```python
from build123d import *

# Parameters (mm, degrees)
SKETCH_1_W          = 250
SKETCH_1_H          = 4
EXTRUDE_1_DEPTH     = 20
EXTRUDE_1_2_DEPTH   = 20
SKETCH_2_W          = 250
SKETCH_2_H          = 28
EXTRUDE_2_DEPTH     = 4
SKETCH_3_W          = 250
SKETCH_3_H          = 4
EXTRUDE_3_DEPTH     = 48.5
EXTRUDE_4_DEPTH     = 250
CUT_EXTRUDE_1_DEPTH = 55
FILLET_1_R          = 2
CUT_EXTRUDE_2_DEPTH = 250


with BuildPart() as part:
    # Sketch 1 → Extrude 1 (new body)
    with BuildSketch(Plane(origin=(0, 0, 0), x_dir=(0, 0, -1), z_dir=(1, 0, 0))):
        with Locations((84.36416185, 14.963552055)):
            Rectangle(SKETCH_1_W, SKETCH_1_H)
    extrude(amount=EXTRUDE_1_DEPTH)



with BuildPart() as body_2:
    # Sketch 1 → Extrude 1 2 (new body)
    with BuildSketch(Plane(origin=(0, 0, 0), x_dir=(0, 0, -1), z_dir=(1, 0, 0))):
        with Locations((84.36416185, -9.036447945)):
            Rectangle(SKETCH_1_W, SKETCH_1_H)
    extrude(amount=EXTRUDE_1_2_DEPTH)


with BuildPart() as part_1:
    add(part.part)

    add(body_2.part)  # Extrude 2 merges body 2
    # Sketch 2 → Extrude 2 (add)
    with BuildSketch(Plane.ZY):
        with Locations((-84.36416185, 2.963552055)):
            Rectangle(SKETCH_2_W, SKETCH_2_H)
    extrude(amount=EXTRUDE_2_DEPTH)

    # Sketch 3 → Extrude 3 (add)
    with BuildSketch(Plane.ZY.offset(4)):
        with Locations((-84.36416185, -9.036447945)):
            Rectangle(SKETCH_3_W, SKETCH_3_H)
    extrude(amount=EXTRUDE_3_DEPTH)

    # Sketch 5 → Extrude 4 (add)
    with BuildSketch(Plane.XY.offset(40.63583815)):
        Polygon((-4, -7.036447945), (-52.5, -7.036447945), (-4, 7.963552055), align=None)
    extrude(amount=-EXTRUDE_4_DEPTH)

    # Sketch 7 → Cut-Extrude 1 (cut)
    with BuildSketch(Plane(origin=(0, 16.963552055, 0), x_dir=(1, 0, 0), z_dir=(0, 1, 0))):
        Polygon((-36.220043801, 209.36416185), (-17.937285277, 177.697495183), (20, 177.697495183), (20, 209.36416185), align=None)
        Polygon((20, 157.697495183), (-22.217241476, 157.697495183), (-40.5, 126.030828516), (-22.217241476, 94.36416185), (20, 94.36416185), align=None)
        Polygon((-40.5, 196.77726344), (-40.5, 146.030828516), (-25.850766068, 171.404045978), align=None)
        Polygon((-40.5, 106.030828516), (-27.990744168, 84.36416185), (-40.5, 84.36416185), align=None)
    cut_extrude_1 = extrude(amount=-CUT_EXTRUDE_1_DEPTH, mode=Mode.SUBTRACT)

    # Mirror 1: Cut-Extrude 1 across plane
    add(cut_extrude_1.mirror(Plane(origin=(0, 0, -84.36416185), x_dir=(1, 0, 0), z_dir=(0, 0, -1))), mode=Mode.SUBTRACT)

    # Fillet 1
    fillet_1_edges = [part_1.edges().sort_by_distance(p)[0] for p in [
        (-22.217241476, -4.353547142, -94.36416185),
        (-40.5, -7.180777842, -126.030828516),
        (-22.217241476, -4.353547142, -157.697495183),
        (-40.5, -7.180777842, -106.030828516),
        (-27.990744168, -5.246356837, -84.36416185),
        (-17.937285277, -3.691698245, -177.697495183),
        (-25.850766068, -4.915432388, 2.675722279),
        (-40.5, -7.180777842, 28.048939741),
        (-40.5, -7.180777842, -22.697495183),
        (-22.217241476, -4.353547142, -11.030828516),
        (-40.5, -7.180777842, -42.697495183),
        (-22.217241476, -4.353547142, -74.36416185),
        (-40.5, -7.180777842, -62.697495183),
        (-17.937285277, -3.691698245, 8.969171484),
        (-40.5, -7.180777842, -196.77726344),
        (-25.850766068, -4.915432388, -171.404045978),
        (-40.5, -7.180777842, -146.030828516),
    ]]
    fillet(fillet_1_edges, radius=FILLET_1_R)

    # Sketch 8 → Cut-Extrude 2 (cut)
    with BuildSketch(Plane(origin=(0, 0, -209.36416185), x_dir=(-1, 0, 0), z_dir=(0, 0, -1))):
        with BuildLine():
            Line((4, 1.064588398), (4, -5.036447945))
            ThreePointArc((4, -5.036447945), (4.585786438, -6.450661507), (6, -7.036447945))
            Line((6, -7.036447945), (25.726684176, -7.036447945))
            ThreePointArc((25.726684176, -7.036447945), (27.704234228, -5.33527196), (26.317623622, -3.125743737))
            Line((26.317623622, -3.125743737), (6.590939446, 2.975292607))
            ThreePointArc((6.590939446, 2.975292607), (4.812961435, 2.674227937), (4, 1.064588398))
        make_face()
    extrude(amount=-CUT_EXTRUDE_2_DEPTH, mode=Mode.SUBTRACT)


solid = part_1.part
```
Model file for the job. Use its own axes, mm. A direction names the side the tool comes from. Coordinates: 2 decimals unless noted, no trailing zeros. Order: outer loops, then holes, each group sorted by start corner. A loop starts at its lowest first (then second) coordinate and runs counter-clockwise, first axis right, second up. Notation, with made-up numbers: (63.25, 14) -> (102.25, 14) arc R10 cw to (102.25, 29) -> close; hole circle Ø9 at (-30.5, 81.5). An arc over 180 degrees is marked (long way). Return JSON: item names as keys, results as strings.
Item 1: Pin check, flat tips, straight feed: P1, Ø5, axis at x = -19, y = -7, coming from the -Z side; P2, Ø5, axis at y = -1.5, z = -65, coming from the +X side; P3, Ø6, axis at x = -8, y = -5.5, coming from the +Z side. Stop position of each tip, or through.
Model answer:
{"P1": "stops at z = -183.87", "P2": "stops at x = -26.18", "P3": "stops at z = 8.97"}
Item 2: Slice it at A-A (z = -160.5). Write the cut outline in (x, y).
Model answer:
{"outline": "(-52.5, -11.04) -> (-40.5, -11.04) -> (-40.5, -3.33) -> (-52.5, -7.04) -> close; (-32.15, -11.04) -> (20, -11.04) -> (20, -7.04) -> (0, -7.04) -> (0, 12.96) -> (20, 12.96) -> (20, 16.96) -> (-4, 16.96) -> (-4, 7.96) -> (-32.15, -0.74) -> close; hole (-26.32, -3.13) arc R2 ccw to (-25.73, -7.04) -> (-6, -7.04) arc R2 ccw to (-4, -5.04) -> (-4, 1.06) arc R2 ccw to (-6.59, 2.98) -> close"}
Item 3: Slice it at D-D (z = -116.5). Write the cut outline in (x, y), then the cut area to 3 significant figures.
Model answer:
{"outline": "(-52.5, -11.04) -> (-35, -11.04) -> (-35, -1.62) -> (-52.5, -7.04) -> close", "area": "117 mm²"}
Item 4: Mould opens along X. For faces 1 (the face through (-40.5, -7, -172)), 2 (the face through (0, 3, -1)), 3 (the face through (10, 12.964, -168)) say: pulls with the +X half, pulls with the -X half, needs draft (parallel to the pull), parting line crosses it, or undercut.
Model answer:
{"face 1": "undercut", "face 2": "pulls with the +X half", "face 3": "needs draft"}
Item 5: 3-axis set-ups, long thin cutter, end or side, ignore diameter. For faces 4 (the face through (-2, 2, -94.364)), 5 (the face through (-16.592, -0.118, -84.604)), 6 (the face through (-40.5, -7, -84)): which of +Z, -Z, +X, -X, +Y, -Y reach the whole face in a straight line?
Model answer:
{"face 4": "+X, +Y, -Y", "face 5": "+Z, -Z", "face 6": "+Y, -Y"}
Item 6: Slice it at C-C (x = 6). Write the cut outline in (y, z).
Model answer:
{"outline": "(-11.04, -177.7) -> (-7.04, -177.7) -> (-7.04, -157.7) -> (-11.04, -157.7) -> close; (-11.04, -94.36) -> (-7.04, -94.36) -> (-7.04, -74.36) -> (-11.04, -74.36) -> close; (-11.04, -11.03) -> (-7.04, -11.03) -> (-7.04, 8.97) -> (-11.04, 8.97) -> close; (12.96, -177.7) -> (16.96, -177.7) -> (16.96, -157.7) -> (12.96, -157.7) -> close; (12.96, -94.36) -> (16.96, -94.36) -> (16.96, -74.36) -> (12.96, -74.36) -> close; (12.96, -11.03) -> (16.96, -11.03) -> (16.96, 8.97) -> (12.96, 8.97) -> close"}
Item 7: Wall check: line 1 along Z through (x, y) = (16, -8); line 2 along Z through (x, y) = (-37, -6.25); line 3 along X through (y, z) = (9.75, -1.5). Give the ranges that are in metal, low to high. Write a range as from..to.
Model answer:
{"line 1": "z = -177.7..-157.7, -94.36..-74.36, -11.03..8.97", "line 2": "z = -209.36..-190.64, -152.17..-132.09, -119.97..-99.89, -68.84..-48.76, -36.64..-16.56, 21.91..40.64", "line 3": "x = -4..0"}
Item 8: Slice it at B-B (y = 10.75). Write the cut outline in (x, z), then the cut area to 3 significant figures.
Model answer:
{"outline": "(-4, -177.7) -> (0, -177.7) -> (0, -157.7) -> (-4, -157.7) -> close; (-4, -94.36) -> (0, -94.36) -> (0, -74.36) -> (-4, -74.36) -> close; (-4, -11.03) -> (0, -11.03) -> (0, 8.97) -> (-4, 8.97) -> close", "area": "240 mm²"}
